from build123d import *

# Parameters (mm, degrees)
F2_R     = 0.8
F4_DEPTH = 6


with BuildPart() as f1:
    # F0 (on Top) → F1 (revolve)
    with BuildSketch(Plane.XY):
        Polygon((26.3, 0), (0, 0), (0, -8), (1.5, -8), (1.5, -5), (26.3, -5), align=None)
    revolve(axis=Axis((13.15, 0, 0), (1, 0, 0)))

    # F2
    f2_edges = [f1.edges().sort_by_distance(p)[0] for p in [
        (0, 8, 0),
    ]]
    fillet(f2_edges, radius=F2_R)

    # F3 (on face) → F4 (cut)
    with BuildSketch(Plane(origin=(0, 0, 0), x_dir=(0, -1, 0), z_dir=(-1, 0, 0))):
        Polygon((1.445, 2.502813), (-1.445, 2.502813), (-2.89, 0), (-1.445, -2.502813), (1.445, -2.502813), (2.89, 0), align=None)
    extrude(amount=-F4_DEPTH, mode=Mode.SUBTRACT)


solid = f1.part
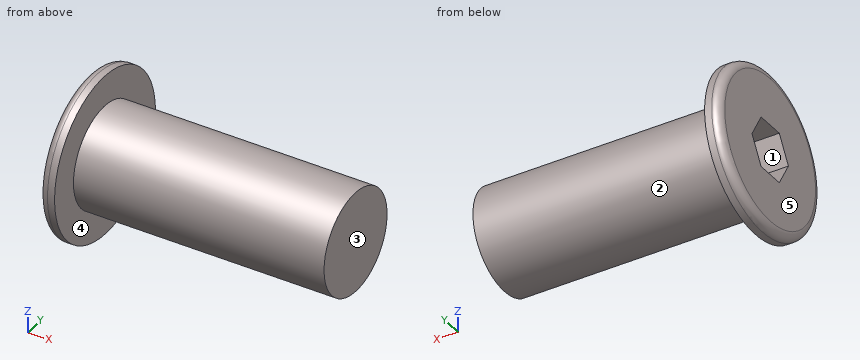
Design review of the part built by this model. Coordinates are the model's own, in mm. Face numbers are marked on the shaded views. A direction names the side the tool comes from. Round coordinates to 2 decimals unless told otherwise and drop trailing zeros. Write each loop counter-clockwise with the first axis right and the second up, starting at its lowest first coordinate (ties: lowest second). Pieces come first, ordered by that corner, then holes.
Item 1: For the marked faces 4 and 5, list the 3-axis set-ups (+Z, -Z, +X, -X, +Y, -Y) from which the entire face can be reached by the end or side of a thin tool; tool diameter is ignored.
Item 2: Wall thickness on L1, parallel to X at y = 1.25, z = -6.75; L2, parallel to Z at x = 3, y = 2.25; L3, parallel to X at y = 0.5, z = 1.5: over which ranges is each line inside the solid? List them lowest first.
Item 3: For pin 1 Ø0.9 at (x, y) = (2.5, -0.5) entering from +Z; pin 2 Ø2 at (x, z) = (9.5, 2) entering from -Y; pin 3 Ø6 at (x, z) = (9.5, 6) entering from +Y, all flat-tipped, find the tip position at first contact; note any pin that passes through.
Item 4: Consider section A-A on y = 0. Give the boundary of the cut face in (x, z).
Item 5: Consider section B-B on x = 24.25. Give the boundary of the cut face in (y, z), and give its area (3 significant figures).
Item 6: Draft analysis for pull direction Z (two halves, no side actions). For the marked faces 1, 2 and 3, state which applies: released by +Z, released by -Z, zero draft, split by the parting line, or undercut.
Check values:
1. face 4: +X
1. face 5: +Z, -Z, -X, +Y, -Y
2. L1: x = 0 to 1.5
2. L2: z = -4.47 to -1.11, 1.11 to 4.47
2. L3: x = 6 to 26.3
3. pin 1: stops at z = 5
3. pin 2: stops at y = -4.9
3. pin 3: stops at y = 4
4. outline: (0, -7.2) arc R0.8 ccw to (0.8, -8) - (1.5, -8) - (1.5, -5) - (26.3, -5) - (26.3, 5) - (1.5, 5) - (1.5, 8) - (0.8, 8) arc R0.8 ccw to (0, 7.2) - (0, 2.5) - (6, 2.5) - (6, -2.5) - (0, -2.5) - close
5. outline: circle Ø10 at (0, 0)
5. area: 78.5 mm2
6. face 1: undercut
6. face 2: split by the parting line
6. face 3: zero draft
